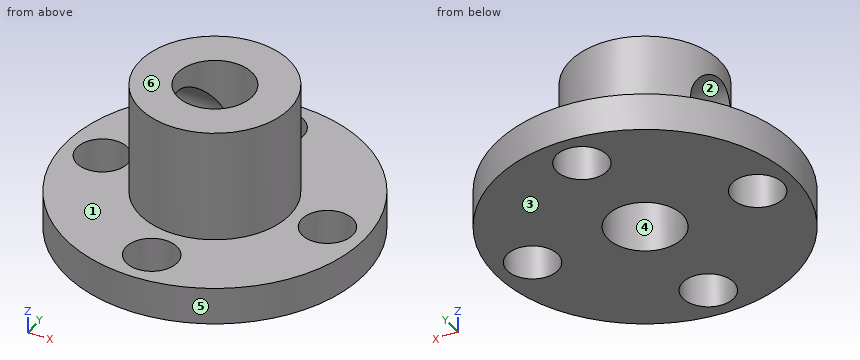
```python
from build123d import *

# Parameters (mm, degrees)
SKETCH2_R           = 12.7
SKETCH2_R_2         = 6.35
SKETCH2_R_3         = 2.159
BOSS_EXTRUDE1_DEPTH = 3.175
SKETCH2_3_R         = 6.35
SKETCH2_3_R_2       = 3.175
BOSS_EXTRUDE2_DEPTH = 12.7
SKETCH4_R           = 3.048
CUT_EXTRUDE1_DEPTH  = 12.7


with BuildPart() as part:
    # Sketch2 → Boss-Extrude1 (new body)
    with BuildSketch(Plane.XY):
        Circle(SKETCH2_R)
        Circle(SKETCH2_R_2, mode=Mode.SUBTRACT)
        with Locations((0, 9.525)):
            Circle(SKETCH2_R_3, mode=Mode.SUBTRACT)
        with Locations((9.525, 0)):
            Circle(SKETCH2_R_3, mode=Mode.SUBTRACT)
        with Locations((0, -9.525)):
            Circle(SKETCH2_R_3, mode=Mode.SUBTRACT)
        with Locations((-9.525, 0)):
            Circle(SKETCH2_R_3, mode=Mode.SUBTRACT)
    extrude(amount=BOSS_EXTRUDE1_DEPTH)

    # Sketch2<3> → Boss-Extrude2 (add)
    with BuildSketch(Plane.XY):
        Circle(SKETCH2_3_R)
        Circle(SKETCH2_3_R_2, mode=Mode.SUBTRACT)
    extrude(amount=BOSS_EXTRUDE2_DEPTH)

    # Sketch4 → Cut-Extrude1 (cut)
    with BuildSketch(Plane(origin=(0, 0, 0), x_dir=(0, 0, -1), z_dir=(1, 0, 0))):
        with Locations((-8.001, 0)):
            Circle(SKETCH4_R)
    extrude(amount=-CUT_EXTRUDE1_DEPTH, mode=Mode.SUBTRACT)


solid = part.part
```
Verification items for the finished model (mm, model axes). Face numbers are marked on the shaded views. A direction names the side the tool comes from. Give positions to 0.01 mm unless a question says otherwise; leave off trailing zeros. Loops run counter-clockwise (first coordinate to the right, second up) from the corner with the lowest first, then second, coordinate; pieces in that order, holes last. Notation, with made-up numbers: M 9,20 L 27,20 A25 cw 27,42 Z; hole C 45,87.5 d3. An arc over 180 degrees is marked long. One line per question, with ' | ' between items.
Item 1: Depth check by flat-ended pin: P1, Ø5, axis at x = -2.5, z = 5.5, coming from the +Y side; P2, Ø3, axis at x = -8.5, y = -9, coming from the +Z side (3 decimals); P3, Ø2, axis at x = -5.5, y = -1.5, coming from the -Z side; P4, Ø5, axis at x = 0, y = 0, coming from the +Z side. Enter the tip coordinate at first touch or a pass-through.
Completed:
P1: stops at y = 12.6 | P2: stops at z = 3.175 | P3: stops at z = 0 | P4: passes through
Item 2: Section check C-C, the plane x = -4.5. Record the cut outline in (y, z) (3 decimals), plus the area to 3 significant figures.
Completed:
outline: M -11.876,0 L 11.876,0 L 11.876,3.175 L 4.48,3.175 L 4.48,12.7 L -4.48,12.7 L -4.48,3.175 L -11.876,3.175 Z; hole C 0,8.001 d6.096 | area: 132 mm^2
Item 3: Section check B-B, the plane y = 0. Record the cut outline in (x, z) (3 decimals).
Completed:
outline: M -12.7,0 L -11.684,0 L -11.684,3.175 L -12.7,3.175 Z; M -7.366,0 L -3.175,0 L -3.175,4.953 L -6.35,4.953 L -6.35,3.175 L -7.366,3.175 Z; M -6.35,11.049 L -3.175,11.049 L -3.175,12.7 L -6.35,12.7 Z; M 3.175,0 L 7.366,0 L 7.366,3.175 L 6.35,3.175 L 6.35,12.7 L 3.175,12.7 Z; M 11.684,0 L 12.7,0 L 12.7,3.175 L 11.684,3.175 Z
Item 4: Thickness scan on line 1 (X direction, y = 0, z = 5) (3 decimals); line 2 (Z direction, x = -1, y = 7.5) (3 decimals); line 3 (Y direction, x = 9.5, z = 1.5). Record the ranges inside material, lowest first. Write a range as [from, to].
Completed:
line 1: x = [3.175, 6.35] | line 2: z = [0, 3.175] | line 3: y = [-8.43, -2.16], [2.16, 8.43]
Item 5: Tool access check on the marked faces 1, 2 and 3. Record the directions out of +Z, -Z, +X, -X, +Y, -Y that give a thin tool (end or side, any length) a straight path to the whole face; none if there is none.
Completed:
face 1: +Z | face 2: -X | face 3: -Z, +X, -X, +Y, -Y
Item 6: Section check A-A, the plane x = 0. Record the cut outline in (y, z) (3 decimals), plus the area to 3 significant figures.
Completed:
outline: M -12.7,0 L -11.684,0 L -11.684,3.175 L -12.7,3.175 Z; M -7.366,0 L -3.175,0 L -3.175,12.7 L -6.35,12.7 L -6.35,3.175 L -7.366,3.175 Z; M 3.175,0 L 7.366,0 L 7.366,3.175 L 6.35,3.175 L 6.35,12.7 L 3.175,12.7 Z; M 11.684,0 L 12.7,0 L 12.7,3.175 L 11.684,3.175 Z | area: 93.5 mm^2
Item 7: Draft check along X on the marked faces 4, 5 and 6. Enter one of: +X half, -X half, draft (parallel to the pull), parting line (faces both ways), or undercut.
Completed:
face 4: undercut | face 5: parting line | face 6: draft
Item 8: Section check D-D, the plane x = -8. Record the cut outline in (y, z) (3 decimals).
Completed:
outline: M -9.864,0 L -1.528,0 L -1.528,3.175 L -9.864,3.175 Z; M 1.528,0 L 9.864,0 L 9.864,3.175 L 1.528,3.175 Z
